from build123d import *

# Parameters (mm, degrees)
SKETCH_2_R          = 4
EXTRUDE_1_DEPTH     = 12
SKETCH_3_R          = 4
CUT_EXTRUDE_1_DEPTH = 20


with BuildPart() as part:
    # 草图2 → 凸台-拉伸1 (new body)
    with BuildSketch(Plane.XY):
        with BuildLine():
            Line((14.282856857, 6), (30, 6))
            Line((30, 6), (30, 8.5))
            Line((30, 8.5), (36, 8.5))
            Line((36, 8.5), (36, 0))
            Line((36, 0), (36, -8.5))
            Line((36, -8.5), (30, -8.5))
            Line((30, -8.5), (30, -6))
            Line((30, -6), (14.282856857, -6))
            ThreePointArc((14.282856857, -6), (11.18447018, -6.624364434), (8.569714114, -8.4))
            ThreePointArc((8.569714114, -8.4), (-12, 0), (8.569714114, 8.4))
            ThreePointArc((8.569714114, 8.4), (11.18447018, 6.624364434), (14.282856857, 6))
        make_face()
        Circle(SKETCH_2_R, mode=Mode.SUBTRACT)
    extrude(amount=EXTRUDE_1_DEPTH)

    # 草图3 → 切除-拉伸1 (cut)
    with BuildSketch(Plane(origin=(36, 0, 0), x_dir=(0, 0, -1), z_dir=(1, 0, 0))):
        with Locations((-6, 0)):
            Circle(SKETCH_3_R)
    extrude(amount=-CUT_EXTRUDE_1_DEPTH, mode=Mode.SUBTRACT)


solid = part.part
Build history of the part. All positions in model axes, mm. A direction names the side the tool comes from. Round coordinates to 2 decimals unless told otherwise and drop trailing zeros. Loops run counter-clockwise (first coordinate to the right, second up) from the corner with the lowest first, then second, coordinate; pieces in that order, holes last. Notation, with made-up numbers: (-39.5, 80) -> (8.5, 80) arc R9 ccw to (8.5, 87) -> close; hole circle Ø5 at (11, 58). An arc over 180 degrees is marked (long way). Answer in a Markdown table with one row per item.
Item 1: Saw through at C-C (y = 0). Write the cut outline in (x, z).
Answers below:
| item | result |
|---|---|
| outline | (-12, 0) -> (-4, 0) -> (-4, 12) -> (-12, 12) -> close; (4, 0) -> (36, 0) -> (36, 2) -> (16, 2) -> (16, 10) -> (36, 10) -> (36, 12) -> (4, 12) -> close |
Item 2: Which spindle directions (+Z, -Z, +X, -X, +Y, -Y) get a long thin tool onto all of the face, cutting with end or side? Do faces 1 (the flat face through (12, 0, 0)), 2 (the cylindrical face through (26.14, -3.905, 6.867)), 3 (the flat face through (30, -7, 6)), 4 (the flat face through (33, 8.5, 6)), 5 (the cylindrical face through (11.143, 6.642, 5.916)). Say none if no direction does.
Answers below:
| item | result |
|---|---|
| face 1 | -Z, +X, -X, +Y, -Y |
| face 2 | +X |
| face 3 | +Z, -Z, -Y |
| face 4 | +Z, -Z, +X, +Y |
| face 5 | +Z, -Z, +Y |
Item 3: Saw through at A-A (x = 0). Write the cut outline in (y, z).
Answers below:
| item | result |
|---|---|
| outline | (-12, 0) -> (-4, 0) -> (-4, 12) -> (-12, 12) -> close; (4, 0) -> (12, 0) -> (12, 12) -> (4, 12) -> close |
Item 4: Drill centre lines: L1, parallel to Y at x = 0, z = 8; L2, parallel to Y at x = 25, z = 6; L3, parallel to X at y = 6.75, z = 8. Where is each one in solid material? Low to high. Write a range as [from, to].
Answers below:
| item | result |
|---|---|
| L1 | y = [-12, -4], [4, 12] |
| L2 | y = [-6, -4], [4, 6] |
| L3 | x = [-9.92, 10.9], [30, 36] |
Item 5: Mould opens along X. For faces 6 (the flat face through (30, 7, 6)), 7 (the flat face through (33, -8.5, 6)), 8 (the flat face through (16, 0, 6)) say: +X half, -X half, draft (parallel to the pull), parting line (faces both ways), or undercut.
Answers below:
| item | result |
|---|---|
| face 6 | undercut |
| face 7 | draft |
| face 8 | +X half |
Item 6: Pin check, flat tips, straight feed: pin 1 (3 mm diameter, centred on x = 34, z = 4.5, fed in from -Y); pin 2 (5 mm diameter, centred on x = 0, y = 0, fed in from -Z); pin 3 (1.5 mm diameter, centred on y = -8.5, z = 3.5, fed in from -X); pin 4 (3 mm diameter, centred on x = 33, z = 6.5, fed in from +Y). Stop position of each tip, or through.
Answers below:
| item | result |
|---|---|
| pin 1 | stops at y = -8.5 |
| pin 2 | passes through |
| pin 3 | stops at x = -9.16 |
| pin 4 | stops at y = 8.5 |
Item 7: Saw through at D-D (x = 22). Write the cut outline in (y, z), and give its area (3 significant figures).
Answers below:
| item | result |
|---|---|
| outline | (-6, 0) -> (6, 0) -> (6, 12) -> (-6, 12) -> close; hole circle Ø8 at (0, 6) |
| area | 93.7 mm² |
Item 8: Saw through at B-B (z = 11.25). Write the cut outline in (x, y).
Answers below:
| item | result |
|---|---|
| outline | (8.57, -8.4) arc R8 cw to (14.28, -6) -> (30, -6) -> (30, -8.5) -> (36, -8.5) -> (36, 8.5) -> (30, 8.5) -> (30, 6) -> (14.28, 6) arc R8 cw to (8.57, 8.4) arc R12 ccw (long way) to start; hole circle Ø8 at (0, 0) |
